Build history of the part. All positions in model axes, mm. A direction names the side the tool comes from. Coordinates: 2 decimals unless noted, no trailing zeros. Loops run counter-clockwise (first coordinate to the right, second up) from the corner with the lowest first, then second, coordinate; pieces in that order, holes last.
Item 1: 3-axis set-ups, long thin cutter, end or side, ignore diameter. For faces 1 (the face through (94, 20, 10)), 2 (the face through (24, 51, 8)), 3 (the face through (24.992, 62.142, 12.619)), 4 (the face through (15, 20, 10)): which of +Z, -Z, +X, -X, +Y, -Y reach the whole face in a straight line?
Item 2: Flat gauge pins, fed straight in: pin 1 (10 mm diameter, centred on y = 37.5, z = 7.5, fed in from -X); pin 2 (10 mm diameter, centred on x = 8.5, z = 7, fed in from +Y); pin 3 (1.5 mm diameter, centred on x = 90.5, y = 36, fed in from +Z); pin 4 (2 mm diameter, centred on y = 31.5, z = 11, fed in from +X). Where does each tip first touch, or does it go through?
Item 3: Cut at B-B (z = 2.75). List the corners of the cut face in (x, y), and give its area (3 significant figures).
Item 4: Drill centre lines: line 1 along X through (y, z) = (15.5, 10); line 2 along Z through (x, y) = (27, 35); line 3 along X through (y, z) = (68.75, 10). Where is each one in solid material? Low to high.
Item 5: Cut at D-D (y = 60). Count the separate pieces of the cut face and the enclosed holes in it, and give its area (3 significant figures).
Item 6: Cut at A-A (x = 9). List the corners of the cut face in (y, z).
Item 7: Mould opens along X. For faces 5 (the face through (27.172, 28.362, 10.547)), 6 (the face through (24, 49, 8)), 7 (the face through (20, 66, 10)) say: released by +X, released by -X, zero draft, split by the parting line, or undercut.
Item 8: Cut at C-C (x = 54). List the corners of the cut face in (y, z), and give its area (4 significant figures).
from build123d import *

# Parameters (mm, degrees)
SCHIZZO1_R                                          = 21.5
ESTRUSIONE_ESTRUSIONE1_DEPTH                        = 20
F_8_2_8_2_DIAMETER_HOLE1_D                          = 8.2
CBORE_FOR_M6_HEX_SOCKET_HEAD_CAP_SCREW1_D           = 6.6
CBORE_FOR_M6_HEX_SOCKET_HEAD_CAP_SCREW1_DEPTH       = 50
CBORE_FOR_M6_HEX_SOCKET_HEAD_CAP_SCREW1_CBORE_D     = 11
CBORE_FOR_M6_HEX_SOCKET_HEAD_CAP_SCREW1_CBORE_DEPTH = 6.4
CBORE_FOR_M6_HEX_SOCKET_HEAD_CAP_SCREW1_TIP         = 1.982840043
SCHIZZO7_W                                          = 15.52137419
SCHIZZO7_H                                          = 2
TAGLIO_ESTRUSIONE1_DEPTH                            = 136.882302012
CHAMFER1_SIZE                                       = 0.5
CHAMFER2_SIZE                                       = 0.5


with BuildPart() as part:
    # Schizzo1 → Estrusione-Estrusione1 (new body)
    with BuildSketch(Plane.XY):
        Polygon((0, 0), (108, 0), (108, 20), (88, 20), (88, 80), (20, 80), (20, 20), (0, 20), align=None)
        with Locations((54, 50)):
            Circle(SCHIZZO1_R, mode=Mode.SUBTRACT)
    extrude(amount=ESTRUSIONE_ESTRUSIONE1_DEPTH)

    # Ø8.2 (8.2) Diameter Hole1 (through all)
    with Locations(Plane(origin=(9, 20, 10), x_dir=(0, 0, 1), z_dir=(0, 1, 0))):
        with Locations((0, 0), (0, 90)):
            Hole(F_8_2_8_2_DIAMETER_HOLE1_D / 2)

    # CBORE for M6 Hex Socket Head Cap Screw1
    with Locations(Plane(origin=(27, 80, 10), x_dir=(0, 0, 1), z_dir=(0, 1, 0))):
        with Locations((0, 0)):
            CounterBoreHole(CBORE_FOR_M6_HEX_SOCKET_HEAD_CAP_SCREW1_D / 2, CBORE_FOR_M6_HEX_SOCKET_HEAD_CAP_SCREW1_CBORE_D / 2, CBORE_FOR_M6_HEX_SOCKET_HEAD_CAP_SCREW1_CBORE_DEPTH, depth=CBORE_FOR_M6_HEX_SOCKET_HEAD_CAP_SCREW1_DEPTH)
            with Locations((0, 0, -(CBORE_FOR_M6_HEX_SOCKET_HEAD_CAP_SCREW1_DEPTH + CBORE_FOR_M6_HEX_SOCKET_HEAD_CAP_SCREW1_TIP / 2))):  # 118° drill point
                Cone(0, CBORE_FOR_M6_HEX_SOCKET_HEAD_CAP_SCREW1_D / 2, CBORE_FOR_M6_HEX_SOCKET_HEAD_CAP_SCREW1_TIP, mode=Mode.SUBTRACT)

    # Schizzo7 → Taglio-Estrusione1 (cut, through all)
    with BuildSketch(Plane(origin=(0, 0, 0), x_dir=(-1, 0, 0), z_dir=(0, 0, -1))):
        with Locations((-27.66540179, 50)):
            Rectangle(SCHIZZO7_W, SCHIZZO7_H)
    extrude(amount=-TAGLIO_ESTRUSIONE1_DEPTH, mode=Mode.SUBTRACT)

    # Chamfer1
    chamfer1_edges = [part.edges().sort_by_distance(p)[0] for p in [
        (54.500135336, 71.494182112, 0),
    ]]
    chamfer(chamfer1_edges, length=CHAMFER1_SIZE)

    # Chamfer2
    chamfer2_edges = [part.edges().sort_by_distance(p)[0] for p in [
        (54.500135336, 28.505817888, 20),
    ]]
    chamfer(chamfer2_edges, length=CHAMFER2_SIZE)


solid = part.part
Filled sheet:
1. face 1: +Z, -Z, +X, +Y
1. face 2: +Z, -Z, -X
1. face 3: +Y
1. face 4: +Z, -Z, -X, +Y
2. pin 1: stops at x = 20
2. pin 2: stops at y = 20
2. pin 3: passes through
2. pin 4: stops at x = 88
3. outline: (0, 0) - (108, 0) - (108, 20) - (88, 20) - (88, 80) - (20, 80) - (20, 51) - (32.52, 51) arc R21.5 cw (long way) to (32.52, 49) - (20, 49) - (20, 20) - (0, 20) - close
3. area: 4,760 mm2
4. line 1: x = 0 to 4.9, 13.1 to 94.9, 103.1 to 108
4. line 2: z = 0 to 6.7, 13.3 to 20
4. line 3: x = 20 to 23.7, 30.3 to 43.48, 64.52 to 88
5. separate pieces: 2
5. enclosed holes: 1
5. area: 564 mm2
6. outline: (0, 0) - (20, 0) - (20, 5.9) - (0, 5.9) - close; (0, 14.1) - (20, 14.1) - (20, 20) - (0, 20) - close
7. face 5: undercut
7. face 6: zero draft
7. face 7: released by -X
8. outline: (0, 0) - (28, 0) - (28.5, 0.5) - (28.5, 19.5) - (28, 20) - (0, 20) - close; (71.5, 0.5) - (72, 0) - (80, 0) - (80, 20) - (72, 20) - (71.5, 19.5) - close
8. area: 739.5 mm2
